from build123d import *

# Parameters (mm, degrees)
SKETCH1_R                        = 5
BOSS_EXTRUDE1_DEPTH              = 15
FILLET1_R                        = 3.175
TAP_DRILL_FOR_M8X1_25_TAP1_D     = 6.8
TAP_DRILL_FOR_M8X1_25_TAP1_DEPTH = 20
TAP_DRILL_FOR_M8X1_25_TAP1_TIP   = 2.042926105


with BuildPart() as part:
    # Sketch1 → Boss-Extrude1 (new body)
    with BuildSketch(Plane.XY):
        with BuildLine():
            Line((-38.1, 4), (-38.1, -4))
            Line((-38.1, -4), (38.1, -4))
            Line((38.1, -4), (38.1, 4))
            Line((38.1, 4), (15, 4))
            Line((15, 4), (15, 12))
            ThreePointArc((15, 12), (0, 27), (-15, 12))
            Line((-15, 12), (-15, 4))
            Line((-15, 4), (-38.1, 4))
        make_face()
        with Locations((0, 12)):
            Circle(SKETCH1_R, mode=Mode.SUBTRACT)
    extrude(amount=BOSS_EXTRUDE1_DEPTH)

    # Fillet1
    fillet1_edges = [part.edges().sort_by_distance(p)[0] for p in [
        (15, 4, 7.5),
        (-15, 4, 7.5),
    ]]
    fillet(fillet1_edges, radius=FILLET1_R)

    # Tap Drill for M8x1.25 Tap1
    with Locations(Plane(origin=(0, 4, 0), x_dir=(1, 0, 0), z_dir=(0, 1, 0))):
        with Locations((29.6, -7.5), (-29.6, -7.5)):
            Hole(TAP_DRILL_FOR_M8X1_25_TAP1_D / 2, depth=TAP_DRILL_FOR_M8X1_25_TAP1_DEPTH)
            with Locations((0, 0, -(TAP_DRILL_FOR_M8X1_25_TAP1_DEPTH + TAP_DRILL_FOR_M8X1_25_TAP1_TIP / 2))):  # 118° drill point
                Cone(0, TAP_DRILL_FOR_M8X1_25_TAP1_D / 2, TAP_DRILL_FOR_M8X1_25_TAP1_TIP, mode=Mode.SUBTRACT)


solid = part.part
CAD build for the part. Positions are in the model's coordinates, mm. A direction names the side the tool comes from. Give positions to 0.01 mm unless a question says otherwise; leave off trailing zeros. Order: outer loops, then holes, each group sorted by start corner. A loop starts at its lowest first (then second) coordinate and runs counter-clockwise, first axis right, second up. Notation, with made-up numbers: (14.5, 63.25) - (35.5, 63.25) arc R19 cw to (35.5, 67.25) - close; hole circle Ø3 at (86, -22.5). An arc over 180 degrees is marked (long way). Answer in a Markdown table with one row per item.
1. Pull direction Y, two halves, no side cores. Call faces 1 (the cylindrical face through (26.46, -0.06, 8.8)), 2 (the cylindrical face through (-0.651, 16.957, 7.395)), 3 (the flat face through (26, 4, 7)): pulls with the +Y half, pulls with the -Y half, needs draft (parallel to the pull), parting line crosses it, or undercut.
Data:
| item | result |
|---|---|
| face 1 | needs draft |
| face 2 | undercut |
| face 3 | pulls with the +Y half |
2. Saw through at D-D, the plane y = 21.5. Give the cut face in (x, z), plus the area to 3 significant figures.
Data:
| item | result |
|---|---|
| outline | (-11.61, 0) - (11.61, 0) - (11.61, 15) - (-11.61, 15) - close |
| area | 348 mm² |
3. Flat gauge pins, fed straight in: pin 1 (8 mm diameter, centred on y = 9.5, z = 6.5, fed in from +X); pin 2 (2 mm diameter, centred on y = 23, z = 8.5, fed in from +X); pin 3 (1 mm diameter, centred on x = -27.5, z = 2, fed in from +Y); pin 4 (8 mm diameter, centred on x = 0, y = 12, fed in from -Z). Where does each tip first touch, or does it go through?
Data:
| item | result |
|---|---|
| pin 1 | stops at x = 15.48 |
| pin 2 | stops at x = 11.18 |
| pin 3 | stops at y = 4 |
| pin 4 | passes through |
4. Saw through at A-A, the plane x = 0. Give the cut face in (y, z), plus the area to 3 significant figures.
Data:
| item | result |
|---|---|
| outline | (-4, 0) - (7, 0) - (7, 15) - (-4, 15) - close; (17, 0) - (27, 0) - (27, 15) - (17, 15) - close |
| area | 315 mm² |
5. Saw through at C-C, the plane y = 8.5. Give the cut face in (x, z), plus the area to 3 significant figures.
Data:
| item | result |
|---|---|
| outline | (-15, 0) - (-3.57, 0) - (-3.57, 15) - (-15, 15) - close; (3.57, 0) - (15, 0) - (15, 15) - (3.57, 15) - close |
| area | 343 mm² |
6. Saw through at B-B, the plane z = 7.5. Give the cut face in (x, y) (3 decimals).
Data:
| item | result |
|---|---|
| outline | (-38.1, -4) - (-33, -4) - (-33, 4) - (-38.1, 4) - close; (-26.2, -4) - (26.2, -4) - (26.2, 4) - (18.175, 4) arc R3.175 cw to (15, 7.175) - (15, 12) arc R15 ccw to (-15, 12) - (-15, 7.175) arc R3.175 cw to (-18.175, 4) - (-26.2, 4) - close; (33, -4) - (38.1, -4) - (38.1, 4) - (33, 4) - close; hole circle Ø10 at (0, 12) |
7. Tool access for faces 4 (the flat face through (-15, 10, 7)), 5 (the flat face through (-1, 5, 15)), 6 (the flat face through (15, 10, 7)): list every direction of +Z, -Z, +X, -X, +Y, -Y with a clear straight run to the whole face (end or side of a thin tool).
Data:
| item | result |
|---|---|
| face 4 | +Z, -Z, -X, +Y |
| face 5 | +Z, +X, -X, +Y, -Y |
| face 6 | +Z, -Z, +X, +Y |
8. Probe probe 1 along X at (y, z) = (2, 10.25); probe 2 along Y at (x, z) = (-34, 10); probe 3 along X at (y, z) = (16.5, 2.75). List the from-to ranges inside material, lowest first. Write a range as [from, to].
Data:
| item | result |
|---|---|
| probe 1 | x = [-38.1, -31.6], [-27.6, 27.6], [31.6, 38.1] |
| probe 2 | y = [-4, 4] |
| probe 3 | x = [-14.31, -2.18], [2.18, 14.31] |
